For this review, take the finished solid that the model builds, in its own axes (mm). A direction names the side the tool comes from. Round coordinates to 2 decimals unless told otherwise and drop trailing zeros. Write each loop counter-clockwise with the first axis right and the second up, starting at its lowest first coordinate (ties: lowest second). Pieces come first, ordered by that corner, then holes. Notation, with made-up numbers: M 46,53 L 75,53 A16 cw 75,63 Z; hole C 30,20.5 d3. An arc over 180 degrees is marked long. Answer in a Markdown table with one row per item.
Autodesk Inventor part; units mm, degrees
ref_plane "YZ Plane" through (0, 0, 0) normal (1, 0, 0) x (0, 1, 0)
ref_plane "XZ Plane" through (0, 0, 0) normal (0, 1, 0) x (-1, 0, 0)
ref_plane "XY Plane" through (0, 0, 0) normal (0, 0, 1) x (1, 0, 0)
sketch "スケッチ1" plane through (0, 0, 0) normal (0, 1, 0) x (-1, 0, 0)
  circle A0 centre (0, 0) radius 18.85
  circle A1 centre (0, 0) radius 14.2
  dimension "d0" = 37.7
  dimension "d1" = 28.4
extrude "押し出し1" add sketch "スケッチ1" along normal blind 15
sketch "スケッチ2" plane through (0, 15, 0) normal (0, 1, 0) x (1, 0, 0)
  circle A0 centre (0, 0) radius 17.15
  dimension "d4" = 34.3
extrude "押し出し2" cut sketch "スケッチ2" against normal blind 14
sketch "スケッチ3" plane through (0, 15, 0) normal (0, 1, 0) x (1, 0, 0)
  circle A0 centre (0, 0) radius 17.15
  circle A1 centre (0, 0) radius 20
  dimension "d7" = 34.3
  dimension "d8" = 40
extrude "押し出し3" add sketch "スケッチ3" along normal blind 2
properties part number "B_pipe_flange_spacer_5" material "ステンレス鋼"
Q1. Machinability: for faces 4 (the face through (-15, 15, -12)), 5 (the face through (-10.2, 1, -10.2)), 6 (the face through (9, 17, -15)), which of the approach directions +Z, -Z, +X, -X, +Y, -Y give a long, thin tool a straight path to every point of the face, cutting with its end or side? Answer none if there is none.
Found:
| item | result |
|---|---|
| face 4 | -Y |
| face 5 | +Y |
| face 6 | +Z, -Z, +X, -X, +Y |
Q2. For probe 1 along Z at (x, y) = (0, 12); probe 2 along Z at (x, y) = (0, 0.4); probe 3 along X at (y, z) = (4.75, -11.5), list the stretches that pass through material, from the lowest coordinate up.
Found:
| item | result |
|---|---|
| probe 1 | -18.85 to -17.15, 17.15 to 18.85 |
| probe 2 | -18.85 to -14.2, 14.2 to 18.85 |
| probe 3 | -14.94 to -12.72, 12.72 to 14.94 |
Q3. Take a section at A-A (x = 0). State the section outline as (y, z) points.
Found:
| item | result |
|---|---|
| outline | M 0,-18.85 L 15,-18.85 L 15,-20 L 17,-20 L 17,-17.15 L 1,-17.15 L 1,-14.2 L 0,-14.2 Z; M 0,14.2 L 1,14.2 L 1,17.15 L 17,17.15 L 17,20 L 15,20 L 15,18.85 L 0,18.85 Z |
Q4. Mouldability with a two-part tool opening along Z and no side actions: class faces 1 (the face through (-2.7, 0, 14.1)), 2 (the face through (16.36, 8.89, 5.15)), 3 (the face through (4.1, 7.4, 18.4)) as +Z half, -Z half, draft (parallel to the pull), parting line (faces both ways), or undercut.
Found:
| item | result |
|---|---|
| face 1 | draft |
| face 2 | undercut |
| face 3 | parting line |
Q5. Take a section at B-B (z = 0). State the section outline as (x, y) points, then the cut area to 3 significant figures.
Found:
| item | result |
|---|---|
| outline | M -20,15 L -18.85,15 L -18.85,0 L -14.2,0 L -14.2,1 L -17.15,1 L -17.15,17 L -20,17 Z; M 14.2,0 L 18.85,0 L 18.85,15 L 20,15 L 20,17 L 17.15,17 L 17.15,1 L 14.2,1 Z |
| area | 68.3 mm² |
Q6. Insertion check: P1, Ø1.5, axis at x = 12, z = -15, coming from the -Y side; P2, Ø2, axis at x = -3.5, y = 6.5, coming from the +Z side; P3, Ø6, axis at x = -11, z = -4.5, coming from the +Y side; P4, Ø5, axis at y = 3, z = -14.5, coming from the +X side. Each pin has a flat end and moves straight along its axis. Give the tip position at first contact, or say it passes through.
Found:
| item | result |
|---|---|
| P1 | y = 0 |
| P2 | z = 18.68 |
| P3 | y = 1 |
| P4 | x = 14.54 |
Q7. Take a section at C-C (y = 14.5). State the section outline as (x, z) points.
Found:
| item | result |
|---|---|
| outline | C 0,0 d37.7; hole C 0,0 d34.3 |
